Build history of the part. All positions in model axes, mm. Face numbers are marked on the shaded views. A direction names the side the tool comes from. Give positions to 0.01 mm unless a question says otherwise; leave off trailing zeros. Loops run counter-clockwise (first coordinate to the right, second up) from the corner with the lowest first, then second, coordinate; pieces in that order, holes last. Notation, with made-up numbers: M 45.25,73.25 L 88.25,73.25 A14 ccw 88.25,96.25 Z; hole C -29.75,81.5 d8. An arc over 180 degrees is marked long. Answer in a Markdown table with one row per item. Add a question column.
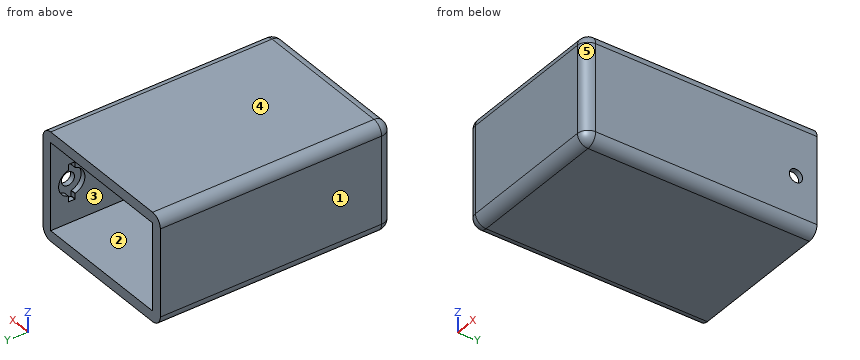
```python
from build123d import *

# Parameters (mm, degrees)
ESBO_O1_W                = 61
ESBO_O1_H                = 92
ESBO_O1_W_2              = 53
ESBO_O1_H_2              = 84
RESSALTO_EXTRUS_O2_DEPTH = 33
ESBO_O5_W                = 61
ESBO_O5_H                = 92
RESSALTO_EXTRUS_O4_DEPTH = 4
ESBO_O6_R                = 2.5
CORTE_EXTRUS_O4_DEPTH    = 4
CORTE_EXTRUS_O5_DEPTH    = 2
ESBO_O8_W                = 61
ESBO_O8_H                = 92
RESSALTO_EXTRUS_O5_DEPTH = 4
ESBO_O9_W                = 61
ESBO_O9_H                = 41
CORTE_EXTRUS_O6_DEPTH    = 4
FILETE1_R                = 4


with BuildPart() as part:
    # Esboço1 → Ressalto-extrusão2 (new body)
    with BuildSketch(Plane.XY):
        with Locations((-12.234044221, -22.462857143)):
            Rectangle(ESBO_O1_W, ESBO_O1_H)
        with Locations((-12.234044221, -22.462857143)):
            Rectangle(ESBO_O1_W_2, ESBO_O1_H_2, mode=Mode.SUBTRACT)
    extrude(amount=-RESSALTO_EXTRUS_O2_DEPTH)

    # Esboço5 → Ressalto-extrusão4 (add)
    with BuildSketch(Plane.XY):
        with Locations((-12.234044221, -22.462857143)):
            Rectangle(ESBO_O5_W, ESBO_O5_H)
    extrude(amount=RESSALTO_EXTRUS_O4_DEPTH)

    # Esboço6 → Corte-extrusão4 (cut)
    with BuildSketch(Plane(origin=(18.265955779, 0, 0), x_dir=(0, 0, -1), z_dir=(1, 0, 0))):
        with Locations((18, 11.537142857)):
            Circle(ESBO_O6_R)
    extrude(amount=-CORTE_EXTRUS_O4_DEPTH, mode=Mode.SUBTRACT)

    # Esboço7 → Corte-extrusão5 (cut)
    with BuildSketch(Plane.ZY.offset(-14.265955779)):
        with BuildLine():
            Line((-11.1, 10.287142857), (-13.081921107, 10.287142857))
            ThreePointArc((-13.081921107, 10.287142857), (-13.142555013, 10.26666348), (-13.178354026, 10.213613445))
            ThreePointArc((-13.178354026, 10.213613445), (-18, 6.537142857), (-22.821645974, 10.213613445))
            ThreePointArc((-22.821645974, 10.213613445), (-22.857444987, 10.26666348), (-22.918078893, 10.287142857))
            Line((-22.918078893, 10.287142857), (-24.9, 10.287142857))
            ThreePointArc((-24.9, 10.287142857), (-24.970710678, 10.316432179), (-25, 10.387142857))
            Line((-25, 10.387142857), (-25, 12.687142857))
            ThreePointArc((-25, 12.687142857), (-24.970710678, 12.757853535), (-24.9, 12.787142857))
            Line((-24.9, 12.787142857), (-22.918078893, 12.787142857))
            ThreePointArc((-22.918078893, 12.787142857), (-22.857444987, 12.807622235), (-22.821645974, 12.860672269))
            ThreePointArc((-22.821645974, 12.860672269), (-18, 16.537142857), (-13.178354026, 12.860672269))
            ThreePointArc((-13.178354026, 12.860672269), (-13.142555013, 12.807622235), (-13.081921107, 12.787142857))
            Line((-13.081921107, 12.787142857), (-11.1, 12.787142857))
            ThreePointArc((-11.1, 12.787142857), (-11.029289322, 12.757853535), (-11, 12.687142857))
            Line((-11, 12.687142857), (-11, 10.387142857))
            ThreePointArc((-11, 10.387142857), (-11.029289322, 10.316432179), (-11.1, 10.287142857))
        make_face()
    extrude(amount=-CORTE_EXTRUS_O5_DEPTH, mode=Mode.SUBTRACT)

    # Esboço8 → Ressalto-extrusão5 (add)
    with BuildSketch(Plane(origin=(0, 0, -33), x_dir=(-1, 0, 0), z_dir=(0, 0, -1))):
        with Locations((12.234044221, -22.462857143)):
            Rectangle(ESBO_O8_W, ESBO_O8_H)
    extrude(amount=RESSALTO_EXTRUS_O5_DEPTH)

    # Esboço9 → Corte-extrusão6 (cut)
    with BuildSketch(Plane(origin=(0, 23.537142857, 0), x_dir=(1, 0, 0), z_dir=(0, 1, 0))):
        with Locations((-12.234044221, 16.5)):
            Rectangle(ESBO_O9_W, ESBO_O9_H)
    extrude(amount=-CORTE_EXTRUS_O6_DEPTH, mode=Mode.SUBTRACT)

    # Filete1
    filete1_edges = [part.edges().sort_by_distance(p)[0] for p in [
        (18.265955779, -24.462857143, -37),
        (-42.734044221, -24.462857143, 4),
        (-12.234044221, -68.462857143, 4),
        (18.265955779, -24.462857143, 4),
        (18.265955779, -68.462857143, -16.5),
        (-42.734044221, -68.462857143, -16.5),
        (-12.234044221, -68.462857143, -37),
        (-42.734044221, -24.462857143, -37),
    ]]
    fillet(filete1_edges, radius=FILETE1_R)


solid = part.part
```
(1) Slice it at A-A, the plane z = -18. Give the cut face in (x, y).
(2) Slice it at B-B, the plane y = -39. Give the cut face in (x, z).
(3) Pin check, flat tips, straight feed: pin 1 (10 mm diameter, centred on x = -12, z = -23, fed in from +Y); pin 2 (1 mm diameter, centred on x = 15.5, y = 12, fed in from +Z); pin 3 (1.6 mm diameter, centred on x = 15.5, y = 11.5, fed in from -Z). Stop position of each tip, or through.
(4) Pull direction Z, two halves, no side cores. Call the marked faces 3, 4 and 5: +Z half, -Z half, draft (parallel to the pull), parting line (faces both ways), or undercut.
(5) Slice it at C-C, the plane z = -29.5. Give the cut face in (x, y).
(6) Tool access for the marked faces 1 and 2: list every direction of +Z, -Z, +X, -X, +Y, -Y with a clear straight run to the whole face (end or side of a thin tool).
(7) Slice it at D-D, the plane x = -25. Give the cut face in (y, z), then the cut area to 3 significant figures.
(8) Wall check: line 1 (X direction, y = -34.5, z = -17); line 2 (Z direction, x = -17, y = -1); line 3 (Y direction, x = -23.5, z = -24.5). Give the ranges that are in metal, low to high.
Solution:
| question | item | result |
|---|---|---|
| 1 | outline | M -42.73,-64.46 A4 ccw -38.73,-68.46 L 14.27,-68.46 A4 ccw 18.27,-64.46 L 18.27,9.04 L 16.27,9.04 L 16.27,6.54 L 14.27,6.54 L 14.27,-64.46 L -38.73,-64.46 L -38.73,19.54 L -42.73,19.54 Z; M 14.27,16.54 L 16.27,16.54 L 16.27,14.04 L 18.27,14.04 L 18.27,19.54 L 14.27,19.54 Z |
| 2 | outline | M -42.73,-33 A4 ccw -38.73,-37 L 14.27,-37 A4 ccw 18.27,-33 L 18.27,0 A4 ccw 14.27,4 L -38.73,4 A4 ccw -42.73,0 Z; hole M -38.73,-33 L 14.27,-33 L 14.27,0 L -38.73,0 Z |
| 3 | pin 1 | y = -64.46 |
| 3 | pin 2 | z = 3.93 |
| 3 | pin 3 | z = -36.98 |
| 4 | face 3 | undercut |
| 4 | face 4 | +Z half |
| 4 | face 5 | draft |
| 5 | outline | M -42.73,-64.46 A4 ccw -38.73,-68.46 L 14.27,-68.46 A4 ccw 18.27,-64.46 L 18.27,19.54 L 14.27,19.54 L 14.27,-64.46 L -38.73,-64.46 L -38.73,19.54 L -42.73,19.54 Z |
| 6 | face 1 | +Z, -Z, -X, +Y, -Y |
| 6 | face 2 | +Y |
| 7 | outline | M -68.46,-33 A4 ccw -64.46,-37 L 19.54,-37 L 19.54,-33 L -64.46,-33 L -64.46,0 L 19.54,0 L 19.54,4 L -64.46,4 A4 ccw -68.46,0 Z |
| 7 | area | 829 mm^2 |
| 8 | line 1 | -42.73 to -38.73, 14.27 to 18.27 |
| 8 | line 2 | -37 to -33, 0 to 4 |
| 8 | line 3 | -68.46 to -64.46 |
